Source: CAD feature listing. Evaluate the final solid. Frame: model axes, mm. A direction names the side the tool comes from. Coordinates: 2 decimals unless noted, no trailing zeros. Loops run counter-clockwise (first coordinate to the right, second up) from the corner with the lowest first, then second, coordinate; pieces in that order, holes last.
from build123d import *

# Parameters (mm, degrees)
EXTRUDE_1_DEPTH     = 4.6
SKETCH_1_R          = 2.625
SKETCH_1_W          = 40.4
SKETCH_1_H          = 4.6
CUT_EXTRUDE_1_DEPTH = 4.6
SKETCH_5_R          = 5.75
EXTRUDE_2_DEPTH     = 7
SKETCH_6_R          = 2.6
EXTRUDE_3_DEPTH     = 0.3
FILLET_2_R          = 4
FILLET_3_R          = 9.2625


with BuildPart() as part:
    # 草图3 → 凸台-拉伸1 (new body)
    with BuildSketch(Plane(origin=(0, 0, 0), x_dir=(1, 0, 0), z_dir=(0, 1, 0))):
        Polygon((-18.5, -28), (40, -28), (40, 28), (-18.5, 28), (-18.5, 36), (-45, 36), (-45, 28), (-45, -28), (-45, -36), (-18.5, -36), align=None)
    extrude(amount=EXTRUDE_1_DEPTH)

    # 草图1 → 切除-拉伸1 (cut)
    with BuildSketch(Plane(origin=(0, 0, 0), x_dir=(1, 0, 0), z_dir=(0, 1, 0))):
        with Locations(Location((-31.75, 20.6375, 0), (0, 0, 90))):
            Circle(SKETCH_1_R)
        with Locations(Location((31.75, 20.6375, 0), (0, 0, 90))):
            Circle(SKETCH_1_R)
        with Locations(Location((31.75, -20.6375, 0), (0, 0, 90))):
            Circle(SKETCH_1_R)
        with Locations(Location((-31.75, -20.6375, 0), (0, 0, 90))):
            Circle(SKETCH_1_R)
        with Locations((-13, -10.4375)):
            Rectangle(SKETCH_1_W, SKETCH_1_H)
        with Locations((-13, 10.4375)):
            Rectangle(SKETCH_1_W, SKETCH_1_H)
        Polygon((-3.25, -26.5375), (-3.25, -14.7375), (18.75, -14.7375), (18.75, -26.5375), (18.75, -29.869530405), (-3.25, -29.869530405), align=None)
        Polygon((-3.25, 14.7375), (18.75, 14.7375), (18.75, 26.5375), (18.75, 29.869530405), (-3.25, 29.869530405), (-3.25, 26.5375), align=None)
    extrude(amount=CUT_EXTRUDE_1_DEPTH, mode=Mode.SUBTRACT)

    # 草图5 → 凸台-拉伸2 (add)
    with BuildSketch(Plane(origin=(0, 4.6, 0), x_dir=(1, 0, 0), z_dir=(0, 1, 0))):
        with Locations(Location((31.75, -20.6375, 0), (0, 0, 90))):
            Circle(SKETCH_5_R)
    extrude_2 = extrude(amount=EXTRUDE_2_DEPTH)

    # 草图6 → 凸台-拉伸3 (add)
    with BuildSketch(Plane(origin=(0, 11.6, 0), x_dir=(1, 0, 0), z_dir=(0, 1, 0))):
        with Locations(Location((31.75, -20.6375, 0), (0, 0, 270))):
            Circle(SKETCH_6_R)
    extrude_3 = extrude(amount=EXTRUDE_3_DEPTH)

    # 圆角2
    fillet_2_edges = [part.edges().sort_by_distance(p)[0] for p in [
        (-3.25, 2.3, -28),
        (18.75, 2.3, -28),
        (40, 2.3, -28),
        (40, 2.3, 28),
        (18.75, 2.3, 28),
        (-3.25, 2.3, 28),
        (18.75, 2.3, -14.7375),
        (18.75, 2.3, 14.7375),
        (-18.5, 2.3, 28),
        (-18.5, 2.3, 36),
        (-45, 2.3, 36),
        (-45, 2.3, -36),
        (-18.5, 2.3, -36),
        (-18.5, 2.3, -28),
    ]]
    fillet(fillet_2_edges, radius=FILLET_2_R - 0.0001)  # a hair under: the kernel refuses the full size

    # 镜向1: 凸台-拉伸2, 凸台-拉伸3 across plane
    add(extrude_2.mirror(Plane(origin=(0, 0, 0), x_dir=(0, 0, 1), z_dir=(1, 0, 0))))
    add(extrude_3.mirror(Plane(origin=(0, 0, 0), x_dir=(0, 0, 1), z_dir=(1, 0, 0))))

    # 圆角3
    fillet_3_edges = [part.edges().sort_by_distance(p)[0] for p in [
        (-3.25, 2.3, -14.7375),
        (-3.25, 2.3, 14.7375),
    ]]
    fillet(fillet_3_edges, radius=FILLET_3_R)


solid = part.part
Q1. Line query: line 1 along Z through (x, y) = (-31.75, 1.25); line 2 along Z through (x, y) = (31.75, 1.75); line 3 along X through (y, z) = (4.25, -23.5). Output: solid intervals per line, ascending.
Q2. Section A-A, the plane x = -31.75. Return the cut outline in (y, z).
Q3. Contact query for flat-ended pins moving along their axis: pin 1 Ø3.5 at (x, y) = (-5, 3.5) entering from +Z; pin 2 Ø2 at (y, z) = (3, -26.5) entering from +X; pin 3 Ø6 at (x, y) = (-21.5, 7.5) entering from -Z; pin 4 Ø6 at (x, z) = (-30.5, 23.5) entering from +Y. Output: stop coordinate, or through.
Q4. Section C-C, the plane y = 2.75. Count the separate pieces of the cut face and the enclosed holes in it, plus the area to 3 significant figures.
Q5. Section B-B, the plane x = 31.75. Return the cut outline in (y, z).
Q6. Section D-D, the plane x = -1. Return the cut outline in (y, z).
Q7. Access query for faces 1 (the cylindrical face through (19.891, 2.332, 26.797)), 2 (the cylindrical face through (-37.363, 8.051, 21.884)), 3 (the flat face through (18.75, 2, -21)). Directions: +Z, -Z, +X, -X, +Y, -Y. A direction counts if a zero-diameter tool reaches every point of the face in a straight line with its end or side. Return the directions, or none.
Derived:
1. line 1: z = -36 to -23.26, -18.01 to -12.74, -8.14 to 8.14, 12.74 to 18.01, 23.26 to 36
1. line 2: z = -28 to -23.26, -18.01 to 18.01, 23.26 to 28
1. line 3: x = -45 to -3.24, 18.75 to 40
2. outline: (0, -36) - (4.6, -36) - (4.6, -23.26) - (0, -23.26) - close; (0, -18.01) - (4.6, -18.01) - (4.6, -12.74) - (0, -12.74) - close; (0, -8.14) - (4.6, -8.14) - (4.6, 8.14) - (0, 8.14) - close; (0, 12.74) - (4.6, 12.74) - (4.6, 14.89) - (11.6, 14.89) - (11.6, 18.04) - (11.9, 18.04) - (11.9, 23.24) - (11.6, 23.24) - (11.6, 26.39) - (4.6, 26.39) - (4.6, 36) - (0, 36) - (0, 23.26) - (4.6, 23.26) - (4.6, 18.01) - (0, 18.01) - close
3. pin 1: stops at z = 27.97
3. pin 2: stops at x = 39.71
3. pin 3: stops at z = -35.99
3. pin 4: stops at y = 11.9
4. separate pieces: 1
4. enclosed holes: 6
4. area: 4,160 mm2
5. outline: (0, -28) - (4.6, -28) - (4.6, -23.26) - (0, -23.26) - close; (0, -18.01) - (4.6, -18.01) - (4.6, 14.89) - (11.6, 14.89) - (11.6, 18.04) - (11.9, 18.04) - (11.9, 23.24) - (11.6, 23.24) - (11.6, 26.39) - (4.6, 26.39) - (4.6, 28) - (0, 28) - (0, 23.26) - (4.6, 23.26) - (4.6, 18.01) - (0, 18.01) - close
6. outline: (0, -17.95) - (4.6, -17.95) - (4.6, -12.74) - (0, -12.74) - close; (0, -8.14) - (4.6, -8.14) - (4.6, 8.14) - (0, 8.14) - close; (0, 12.74) - (4.6, 12.74) - (4.6, 17.95) - (0, 17.95) - close
7. face 1: +Z, +Y, -Y
7. face 2: +Y
7. face 3: -Z, +Y, -Y
